Model file for the job. Use its own axes, mm. Round coordinates to 2 decimals unless told otherwise and drop trailing zeros. Loops run counter-clockwise (first coordinate to the right, second up) from the corner with the lowest first, then second, coordinate; pieces in that order, holes last. Notation, with made-up numbers: M -18.5,49.25 L 9.5,49.25 A19 ccw 9.5,75.25 Z; hole C 88.5,1.5 d2. An arc over 180 degrees is marked long. Answer in a Markdown table with one row per item.
from build123d import *

# Parameters (mm, degrees)
SKETCH1_R            = 65.4
BOSS_EXTRUDE1_DEPTH  = 1.5
M6_CLEARANCE_HOLE1_D = 6.6
CIRPATTERN2_COUNT    = 4
M4_CLEARANCE_HOLE1_D = 4.3
CIRPATTERN1_COUNT    = 4
SKETCH10_R           = 7.5
CUT_EXTRUDE1_DEPTH   = 93.538208325
SKETCH11_R           = 2.25
CUT_EXTRUDE2_DEPTH   = 93.538208325


with BuildPart() as part:
    # Sketch1 → Boss-Extrude1 (new, symmetric)
    with BuildSketch(Plane(origin=(0, 0, 0), x_dir=(1, 0, 0), z_dir=(0, 1, 0))):
        with Locations(Location((0, 0, 0), (0, 0, 270))):
            Circle(SKETCH1_R)
    extrude(amount=BOSS_EXTRUDE1_DEPTH, both=True)

    # M6 Clearance Hole1 (through all)
    with Locations(Plane(origin=(0, 1.5, 0), x_dir=(1, 0, 0), z_dir=(0, 1, 0))):
        with Locations((55.4, 0)):
            m6_clearance_hole1 = Hole(M6_CLEARANCE_HOLE1_D / 2)

    # CirPattern2: M6 Clearance Hole1 ×4 about axis
    cirpattern2_axis = Axis((0, 0, 0), (0, 1, 0))
    for i in range(1, CIRPATTERN2_COUNT):
        add(m6_clearance_hole1.rotate(cirpattern2_axis, i * 360 / CIRPATTERN2_COUNT), mode=Mode.SUBTRACT)

    # M4 Clearance Hole1 (through all)
    with Locations(Plane(origin=(0, 1.5, 0), x_dir=(1, 0, 0), z_dir=(0, 1, 0))):
        with Locations((39.173715678, 39.173715678)):
            m4_clearance_hole1 = Hole(M4_CLEARANCE_HOLE1_D / 2)

    # CirPattern1: M4 Clearance Hole1 ×4 about axis
    cirpattern1_axis = Axis((0, 0, 0), (0, 1, 0))
    for i in range(1, CIRPATTERN1_COUNT):
        add(m4_clearance_hole1.rotate(cirpattern1_axis, i * 360 / CIRPATTERN1_COUNT), mode=Mode.SUBTRACT)

    # Sketch10 → Cut-Extrude1 (cut, through all)
    with BuildSketch(Plane(origin=(0, 1.5, 0), x_dir=(1, 0, 0), z_dir=(0, 1, 0))):
        with Locations(Location((0, 0, 0), (0, 0, 270))):
            Circle(SKETCH10_R)
    extrude(amount=-CUT_EXTRUDE1_DEPTH, mode=Mode.SUBTRACT)

    # Sketch11 → Cut-Extrude2 (cut, through all)
    with BuildSketch(Plane.XZ.offset(1.5)):
        with Locations(Location((-14.75, -5, 0), (0, 0, 270))):
            Circle(SKETCH11_R)
        with Locations(Location((-14.75, 5, 0), (0, 0, 270))):
            Circle(SKETCH11_R)
        with Locations(Location((34.75, -5, 0), (0, 0, 270))):
            Circle(SKETCH11_R)
        with Locations(Location((34.75, 5, 0), (0, 0, 270))):
            Circle(SKETCH11_R)
    extrude(amount=-CUT_EXTRUDE2_DEPTH, mode=Mode.SUBTRACT)


solid = part.part
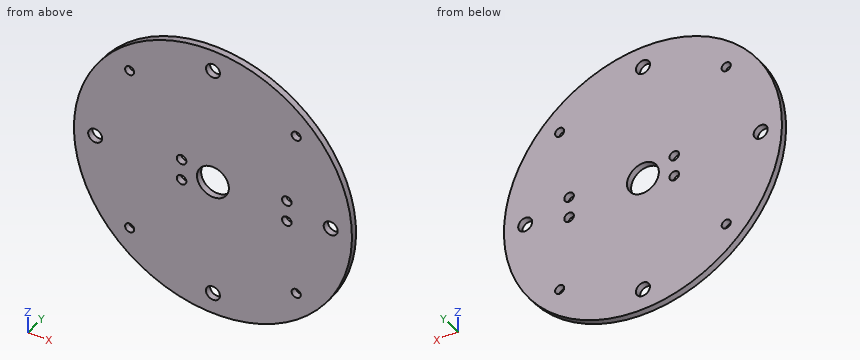
1. Pin check, flat tips, straight feed: pin 1 (1 mm diameter, centred on y = 0, z = -33, fed in from -X); pin 2 (1 mm diameter, centred on x = 50.5, y = -0.5, fed in from +Z). Stop position of each tip, or through.
Verdict:
| item | result |
|---|---|
| pin 1 | stops at x = -56.75 |
| pin 2 | stops at z = 42.16 |
2. Saw through at B-B (x = -14.75). Write the cut outline in (y, z).
Verdict:
| item | result |
|---|---|
| outline | M -1.5,-63.71 L 1.5,-63.71 L 1.5,-7.25 L -1.5,-7.25 Z; M -1.5,-2.75 L 1.5,-2.75 L 1.5,2.75 L -1.5,2.75 Z; M -1.5,7.25 L 1.5,7.25 L 1.5,63.71 L -1.5,63.71 Z |
3. Wall check: probe 1 along Z at (x, y) = (-39.5, 0.75); probe 2 along X at (y, z) = (0.9, 6); probe 3 along X at (y, z) = (0.95, 4). Give the ranges that are in metal, low to high.
Verdict:
| item | result |
|---|---|
| probe 1 | z = -52.12 to -41.3, -37.05 to 37.05, 41.3 to 52.12 |
| probe 2 | x = -65.12 to -16.77, -12.73 to -4.5, 4.5 to 32.73, 36.77 to 65.12 |
| probe 3 | x = -65.28 to -16.77, -12.73 to -6.34, 6.34 to 32.73, 36.77 to 65.28 |
4. Saw through at C-C (z = -5). Write the cut outline in (x, y), and give its area (3 significant figures).
Verdict:
| item | result |
|---|---|
| outline | M -65.21,-1.5 L -17,-1.5 L -17,1.5 L -65.21,1.5 Z; M -12.5,-1.5 L -5.59,-1.5 L -5.59,1.5 L -12.5,1.5 Z; M 5.59,-1.5 L 32.5,-1.5 L 32.5,1.5 L 5.59,1.5 Z; M 37,-1.5 L 65.21,-1.5 L 65.21,1.5 L 37,1.5 Z |
| area | 331 mm² |
5. Saw through at D-D (x = -55.4). Write the cut outline in (y, z), and give its area (3 significant figures).
Verdict:
| item | result |
|---|---|
| outline | M -1.5,-34.76 L 1.5,-34.76 L 1.5,-3.3 L -1.5,-3.3 Z; M -1.5,3.3 L 1.5,3.3 L 1.5,34.76 L -1.5,34.76 Z |
| area | 189 mm² |
6. Saw through at A-A (z = -57). Write the cut outline in (x, y), and give its area (3 significant figures).
Verdict:
| item | result |
|---|---|
| outline | M -32.06,-1.5 L -2.89,-1.5 L -2.89,1.5 L -32.06,1.5 Z; M 2.89,-1.5 L 32.06,-1.5 L 32.06,1.5 L 2.89,1.5 Z |
| area | 175 mm² |
